Verification items for the finished model (mm, model axes). A direction names the side the tool comes from. Coordinates: 2 decimals unless noted, no trailing zeros. Write each loop counter-clockwise with the first axis right and the second up, starting at its lowest first coordinate (ties: lowest second). Pieces come first, ordered by that corner, then holes. Notation, with made-up numbers: (-17.5, -7) -> (8.5, -7) arc R7 ccw to (8.5, 5) -> close; hole circle Ø6 at (27, 55). An arc over 180 degrees is marked (long way). Answer in a Markdown table with one row per item.
```python
from build123d import *

# Parameters (mm, degrees)
SKETCH_1_W          = 40
SKETCH_1_H          = 90
EXTRUDE_1_DEPTH     = 15
CUT_EXTRUDE_1_DEPTH = 100.624294226


with BuildPart() as part:
    # 草图1 → 凸台-拉伸1 (new body)
    with BuildSketch(Plane.XY):
        with Locations((20, -45)):
            Rectangle(SKETCH_1_W, SKETCH_1_H)
    extrude(amount=EXTRUDE_1_DEPTH)

    # 草图2 → 切除-拉伸1 (cut, through all)
    with BuildSketch(Plane.XZ.offset(90)):
        Polygon((10, 15), (7, 10), (33, 10), (30, 15), align=None)
    extrude(amount=-CUT_EXTRUDE_1_DEPTH, mode=Mode.SUBTRACT)


solid = part.part
```
1. Thickness scan on line 1 (Z direction, x = 28, y = -72.5); line 2 (X direction, y = -67.5, z = 12.5); line 3 (Z direction, x = 9, y = -16). Record the ranges inside material, lowest first. Write a range as from..to.
Geometry says:
| item | result |
|---|---|
| line 1 | 0..10 |
| line 2 | 0..8.5, 31.5..40 |
| line 3 | 0..10, 13.33..15 |
2. Section check C-C, the plane x = 13. Record the boundary of the cut face in (y, z), plus the area to 3 significant figures.
Geometry says:
| item | result |
|---|---|
| outline | (-90, 0) -> (0, 0) -> (0, 10) -> (-90, 10) -> close |
| area | 900 mm^2 |
3. Mould release check, pull along X, two halves, no side actions. Record for faces 3 (the flat face through (40, -46, 7)), 4 (the flat face through (20, -46, 10)), 5 (the flat face through (20, -90, 6)), 6 (the flat face through (0, -46, 7)): released by +X, released by -X, zero draft, split by the parting line, or undercut.
Geometry says:
| item | result |
|---|---|
| face 3 | released by +X |
| face 4 | undercut |
| face 5 | zero draft |
| face 6 | released by -X |
4. Section check A-A, the plane x = 8. Record the boundary of the cut face in (y, z), plus the area to 3 significant figures.
Geometry says:
| item | result |
|---|---|
| outline | (-90, 0) -> (0, 0) -> (0, 10) -> (-90, 10) -> close; (-90, 11.67) -> (0, 11.67) -> (0, 15) -> (-90, 15) -> close |
| area | 1,200 mm^2 |
5. Section check B-B, the plane y = -10.5. Record the boundary of the cut face in (x, z), plus the area to 3 significant figures.
Geometry says:
| item | result |
|---|---|
| outline | (0, 0) -> (40, 0) -> (40, 15) -> (30, 15) -> (33, 10) -> (7, 10) -> (10, 15) -> (0, 15) -> close |
| area | 485 mm^2 |
6. Depth check by flat-ended pin: P1, Ø2, axis at x = 20.5, y = -77, coming from the +Z side. Enter the tip coordinate at first touch or a pass-through.
Geometry says:
| item | result |
|---|---|
| P1 | z = 10 |
7. Tool access check on faces 1 (the flat face through (5, -44, 15)), 2 (the flat face through (8.5, -45.6, 12.5)). Record the directions out of +Z, -Z, +X, -X, +Y, -Y that give a thin tool (end or side, any length) a straight path to the whole face; none if there is none.
Geometry says:
| item | result |
|---|---|
| face 1 | +Z, +X, -X, +Y, -Y |
| face 2 | +Y, -Y |
